Design review of the part shown in the three views and the two pictorial views. Dimensions are in mm from the part's minimum x, y and z. A direction names the side the tool comes from. Round coordinates to 2 decimals unless told otherwise and drop trailing zeros. Order: outer loops, then holes, each group sorted by start corner. A loop starts at its lowest first (then second) coordinate and runs counter-clockwise, first axis right, second up. Notation, with made-up numbers: M 16,89.5 L 74,89.5 A22 ccw 74,111.5 Z; hole C 9,-16.75 d2. An arc over 180 degrees is marked long. Write each question's results on one line, items separated by ' | '. Start each with the question number.
Item 1: The part is to be moulded in two halves that separate along X. For the marked faces 3, 4, 5 and 6, say which applies: +X half, -X half, draft (parallel to the pull), parting line (faces both ways), or undercut.
Item 2: Take a section at C-C, the plane y = 10. Write out the cut boundary in (x, z).
Item 3: Machinability: for the marked faces 1 and 2, which of the approach directions +Z, -Z, +X, -X, +Y, -Y give a long, thin tool a straight path to every point of the face, cutting with its end or side? Answer none if there is none.
Item 4: Take a section at A-A, the plane x = 99. Write out the cut boundary in (y, z), plus the area to 3 significant figures.
Item 5: Take a section at B-B, the plane z = 10.5. Write out the cut boundary in (x, y) (1 decimal).
Item 6: Wall thickness on line 1 (Y direction, x = 109, z = 7.5); line 2 (Z direction, x = 7.5, y = 3.5): over which ranges is each line inside the solid? List them lowest first. Write a range as [from, to].
Item 7: Take a section at D-D, the plane z = 36. Write out the cut boundary in (x, y), plus the area to 3 significant figures.
Item 8: Clearance check with flat-ended pins moving along their axes: pin 1 (5 mm diameter, centred on x = 85.5, z = 37, fed in from -Y); pin 2 (12 mm diameter, centred on y = 10, z = 19, fed in from +X). State where each tip first meets the part, or that it passes through.
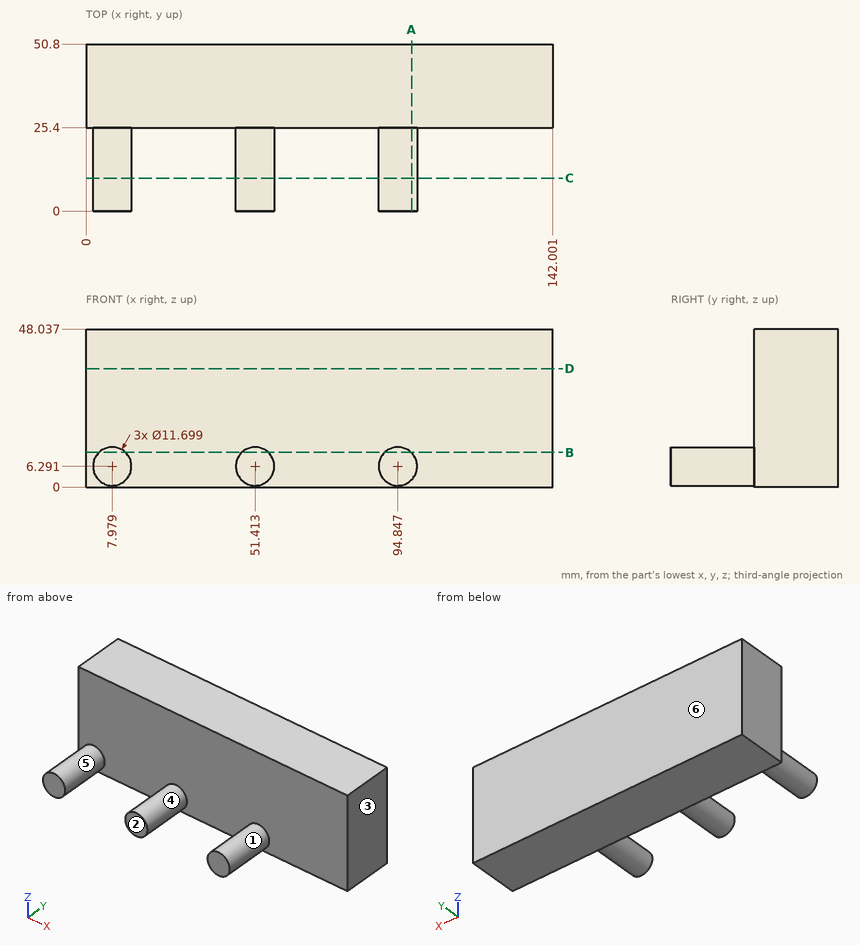
Results list:
1) face 3: +X half | face 4: undercut | face 5: undercut | face 6: draft
2) outline: C 7.98,6.29 d11.7; C 51.41,6.29 d11.7; C 94.85,6.29 d11.7
3) face 1: -Y | face 2: +Z, -Z, +X, -X, -Y
4) outline: M 0,2.17 L 25.4,2.17 L 25.4,0 L 50.8,0 L 50.8,48.04 L 25.4,48.04 L 25.4,10.41 L 0,10.41 Z | area: 1,430 mm²
5) outline: M 0,25.4 L 3.9,25.4 L 3.9,0 L 12,0 L 12,25.4 L 47.4,25.4 L 47.4,0 L 55.5,0 L 55.5,25.4 L 90.8,25.4 L 90.8,0 L 98.9,0 L 98.9,25.4 L 142,25.4 L 142,50.8 L 0,50.8 Z
6) line 1: [25.4, 50.8] | line 2: [0.46, 12.12]
7) outline: M 0,25.4 L 142,25.4 L 142,50.8 L 0,50.8 Z | area: 3,610 mm²
8) pin 1: y = 25.4 | pin 2: through
